from build123d import *

# Parameters (mm, degrees)
BOSS_EXTRUDE1_DEPTH = 2.5
SKETCH2_R           = 1.5
CUT_EXTRUDE1_DEPTH  = 3.5


with BuildPart() as part:
    # Sketch1 → Boss-Extrude1 (new body)
    with BuildSketch(Plane(origin=(0, 0, 0), x_dir=(1, 0, 0), z_dir=(0, 1, 0))):
        with BuildLine():
            Line((10, 0), (120, 0))
            ThreePointArc((120, 0), (127.071067812, 2.928932188), (130, 10))
            Line((130, 10), (130, 45))
            ThreePointArc((130, 45), (127.071067812, 52.071067812), (120, 55))
            Line((120, 55), (10, 55))
            ThreePointArc((10, 55), (2.928932188, 52.071067812), (0, 45))
            Line((0, 45), (0, 10))
            ThreePointArc((0, 10), (2.928932188, 2.928932188), (10, 0))
        make_face()
    extrude(amount=BOSS_EXTRUDE1_DEPTH)

    # Sketch2 → Cut-Extrude1 (cut, through all)
    with BuildSketch(Plane(origin=(0, 2.5, 0), x_dir=(1, 0, 0), z_dir=(0, 1, 0))):
        with Locations((14, 5)):
            Circle(SKETCH2_R)
        with Locations((14, 50)):
            Circle(SKETCH2_R)
        with Locations((116, 5)):
            Circle(SKETCH2_R)
        with Locations((116, 50)):
            Circle(SKETCH2_R)
    extrude(amount=-CUT_EXTRUDE1_DEPTH, mode=Mode.SUBTRACT)


solid = part.part
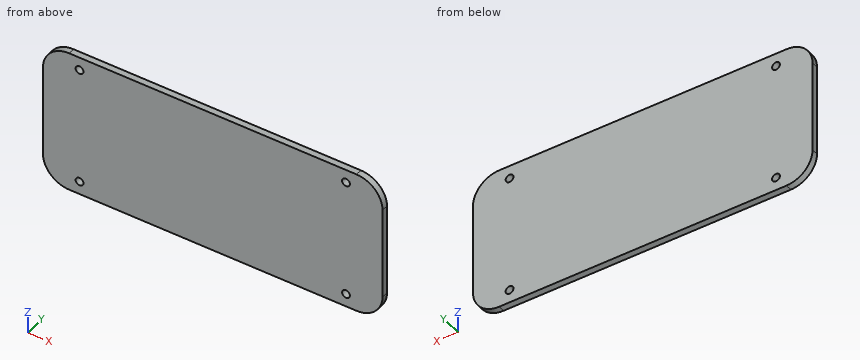
Read the model definition and answer for the solid it produces. Units are mm, in the model's axes. Give positions to 0.01 mm unless a question says otherwise; leave off trailing zeros. Write each loop counter-clockwise with the first axis right and the second up, starting at its lowest first coordinate (ties: lowest second). Pieces come first, ordered by that corner, then holes. Notation, with made-up numbers: (27.5, -22.75) -> (42.5, -22.75) arc R16 cw to (42.5, 1.25) -> close; hole circle Ø5 at (-32.75, 15). An arc over 180 degrees is marked (long way). Answer as a JSON object with one key per item and string values. Group by question number.
1) Find section A-A (z = -5). Write down the section's boundary in (x, y).
2) Find section B-B (x = 14). Write down the section's boundary in (y, z).
3) This flat-tipped pin is pushed along its axis until it touches: P1, Ø10, axis at x = 32.5, z = -14.5, coming from the -Y side. Where does it stop, or does it pass through?
4) Consider L1, parallel to Z at x = 14, y = 1.8; L2, parallel to X at y = 0.55, z = -50; L3, parallel to X at y = 0.35, z = -49. Determine where each line is inside the solid, lowest interval first. Write a range as from..to.
5) Find section C-C (y = 1.85). Write down the section's boundary in (x, z), and give its area (3 significant figures).
Values follow:
{
 "1": {"outline": "(1.34, 0) -> (12.5, 0) -> (12.5, 2.5) -> (1.34, 2.5) -> close; (15.5, 0) -> (114.5, 0) -> (114.5, 2.5) -> (15.5, 2.5) -> close; (117.5, 0) -> (128.66, 0) -> (128.66, 2.5) -> (117.5, 2.5) -> close"},
 "2": {"outline": "(0, -55) -> (2.5, -55) -> (2.5, -51.5) -> (0, -51.5) -> close; (0, -48.5) -> (2.5, -48.5) -> (2.5, -6.5) -> (0, -6.5) -> close; (0, -3.5) -> (2.5, -3.5) -> (2.5, 0) -> (0, 0) -> close"},
 "3": {"P1": "stops at y = 0"},
 "4": {"L1": "z = -55..-51.5, -48.5..-6.5, -3.5..0", "L2": "x = 1.34..12.5, 15.5..114.5, 117.5..128.66", "L3": "x = 0.83..12.88, 15.12..114.88, 117.12..129.17"},
 "5": {"outline": "(0, -45) arc R10 ccw to (10, -55) -> (120, -55) arc R10 ccw to (130, -45) -> (130, -10) arc R10 ccw to (120, 0) -> (10, 0) arc R10 ccw to (0, -10) -> close; hole circle Ø3 at (14, -50); hole circle Ø3 at (14, -5); hole circle Ø3 at (116, -50); hole circle Ø3 at (116, -5)", "area": "7,040 mm2"}
}
